Build history of the part. All positions in model axes, mm. Round coordinates to 2 decimals unless told otherwise and drop trailing zeros. Order: outer loops, then holes, each group sorted by start corner. A loop starts at its lowest first (then second) coordinate and runs counter-clockwise, first axis right, second up. Notation, with made-up numbers: (5.5, -20.5) -> (45.5, -20.5) arc R21 cw to (45.5, 2.5) -> close; hole circle Ø6 at (-30, 80.25). An arc over 180 degrees is marked (long way). Answer as a JSON object with one key per item and string values.
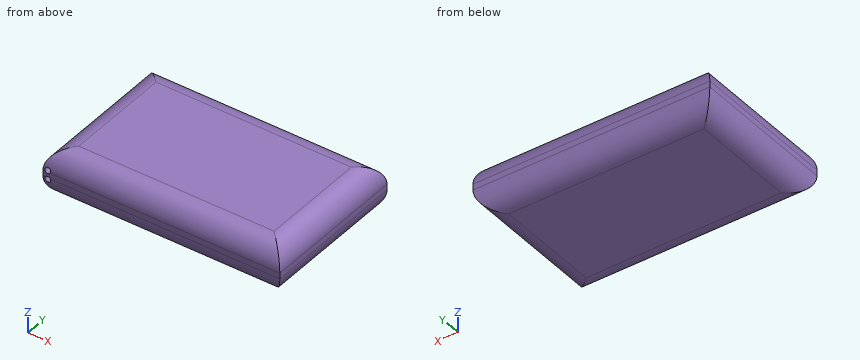
from build123d import *

# Parameters (mm, degrees)
ESBO_O1_W                = 40
ESBO_O1_H                = 25
RESSALTO_EXTRUS_O1_DEPTH = 8
FILETE1_R                = 3.5
ESBO_O2_R                = 0.5
CORTE_EXTRUS_O1_DEPTH    = 2


with BuildPart() as part:
    # Esboço1 → Ressalto-extrusão1 (new body)
    with BuildSketch(Plane.XY):
        Rectangle(ESBO_O1_W, ESBO_O1_H)
    extrude(amount=RESSALTO_EXTRUS_O1_DEPTH)

    # Filete1
    filete1_edges = [part.edges().sort_by_distance(p)[0] for p in [
        (-20, 0, 8),
        (0, -12.5, 8),
        (20, 0, 8),
        (0, -12.5, 0),
        (-20, 0, 0),
        (0, 12.5, 0),
        (20, 0, 0),
        (0, 12.5, 8),
    ]]
    fillet(filete1_edges, radius=FILETE1_R)

    # Esboço2 → Corte-extrusão1 (cut)
    with BuildSketch(Plane.XZ.offset(12.5)):
        with Locations(Location((-19.2, 4.75, 0), (0, 0, 270))):
            Circle(ESBO_O2_R)
        with Locations(Location((-19.2, 3.25, 0), (0, 0, 30))):
            Circle(ESBO_O2_R)
    extrude(amount=-CORTE_EXTRUS_O1_DEPTH, mode=Mode.SUBTRACT)


solid = part.part
1) Cut at A-A, the plane y = 7.25. Give the cut face in (x, z), plus the area to 3 significant figures.
Checked values:
{"outline": "(-20, 3.5) arc R3.5 ccw to (-16.5, 0) -> (16.5, 0) arc R3.5 ccw to (20, 3.5) -> (20, 4.5) arc R3.5 ccw to (16.5, 8) -> (-16.5, 8) arc R3.5 ccw to (-20, 4.5) -> close", "area": "309 mm²"}
2) Flat gauge pin, fed straight in: pin 1 Ø0.5 at (x, z) = (-19, 3) entering from -Y. Where does the tip first touch, or does it go through?
Checked values:
{"pin 1": "stops at y = -12.47"}
3) Cut at D-D, the plane x = -19.2. Give the cut face in (y, z).
Checked values:
{"outline": "(-12.5, 3.75) -> (-10.5, 3.75) -> (-10.5, 2.75) -> (-12.42, 2.75) arc R3.5 ccw to (-11.7, 1.27) -> (11.7, 1.27) arc R3.5 ccw to (12.5, 3.5) -> (12.5, 4.5) arc R3.5 ccw to (11.7, 6.73) -> (-11.7, 6.73) arc R3.5 ccw to (-12.42, 5.25) -> (-10.5, 5.25) -> (-10.5, 4.25) -> (-12.5, 4.25) -> close"}
4) Probe L1, parallel to Z at x = -19.2, y = -11.15; L2, parallel to X at y = -11, z = 4.75; L3, parallel to X at y = 2, z = 4.75. List the from-to ranges inside material, lowest first. Write a range as from..to.
Checked values:
{"L1": "z = 1.27..2.75, 3.75..4.25, 5.25..6.73", "L2": "x = -19.99..-19.7, -18.7..19.99", "L3": "x = -19.99..19.99"}
5) Cut at C-C, the plane z = 6.5. Give the cut face in (x, y).
Checked values:
{"outline": "(-19.37, -11.87) -> (19.37, -11.87) -> (19.37, 11.87) -> (-19.37, 11.87) -> close"}
6) Cut at B-B, the plane x = 13.5. Give the cut face in (y, z), plus the area to 3 significant figures.
Checked values:
{"outline": "(-12.5, 3.5) arc R3.5 ccw to (-9, 0) -> (9, 0) arc R3.5 ccw to (12.5, 3.5) -> (12.5, 4.5) arc R3.5 ccw to (9, 8) -> (-9, 8) arc R3.5 ccw to (-12.5, 4.5) -> close", "area": "189 mm²"}
